Check sheet for the drawn part. Datum: minimum x, y, z corner. Units: mm. A direction names the side the tool comes from. Give positions to 0.01 mm unless a question says otherwise; leave off trailing zeros. Write each loop counter-clockwise with the first axis right and the second up, starting at its lowest first coordinate (ties: lowest second). Pieces come first, ordered by that corner, then holes. Notation, with made-up numbers: (66, -29) - (89, -29) arc R23 cw to (89, -14) - close; hole circle Ø9 at (6, 2). An arc over 180 degrees is marked (long way). Answer as a JSON object with one key per item and string values. Group by question number.
Item 1: Sectioned sample at A-A, the plane z = 16.5. Record the boundary of the cut face in (x, y).
Item 2: Sectioned sample at C-C, the plane z = 5.25. Record the boundary of the cut face in (x, y).
Item 3: Tool access check on the marked faces 1 and 2. Record the directions out of +Z, -Z, +X, -X, +Y, -Y that give a thin tool (end or side, any length) a straight path to the whole face; none if there is none.
Item 4: Draft check along Y on the marked faces 3, 4 and 5. Enter one of: +Y half, -Y half, draft (parallel to the pull), parting line (faces both ways), or undercut.
Item 5: Sectioned sample at B-B, the plane z = 9.5. Record the boundary of the cut face in (x, y).
Item 6: Go/stop test with flat-tipped pins: pin 1 (12 mm diameter, centred on x = 9.5, z = 3.5, fed in from -Y); pin 2 (12 mm diameter, centred on y = 35.5, z = 20.5, fed in from +X); pin 3 (1.5 mm diameter, centred on y = 30, z = 4, fed in from -X). Record where each tip stops, or that it passes through.
Item 7: Scan lines: line 1 along Y through (x, z) = (18.5, 19); line 2 along Y through (x, z) = (25, 20.5); line 3 along Z through (x, y) = (27.5, 6). Record each from-to range of solid material in increasing order. Write a range as [from, to].
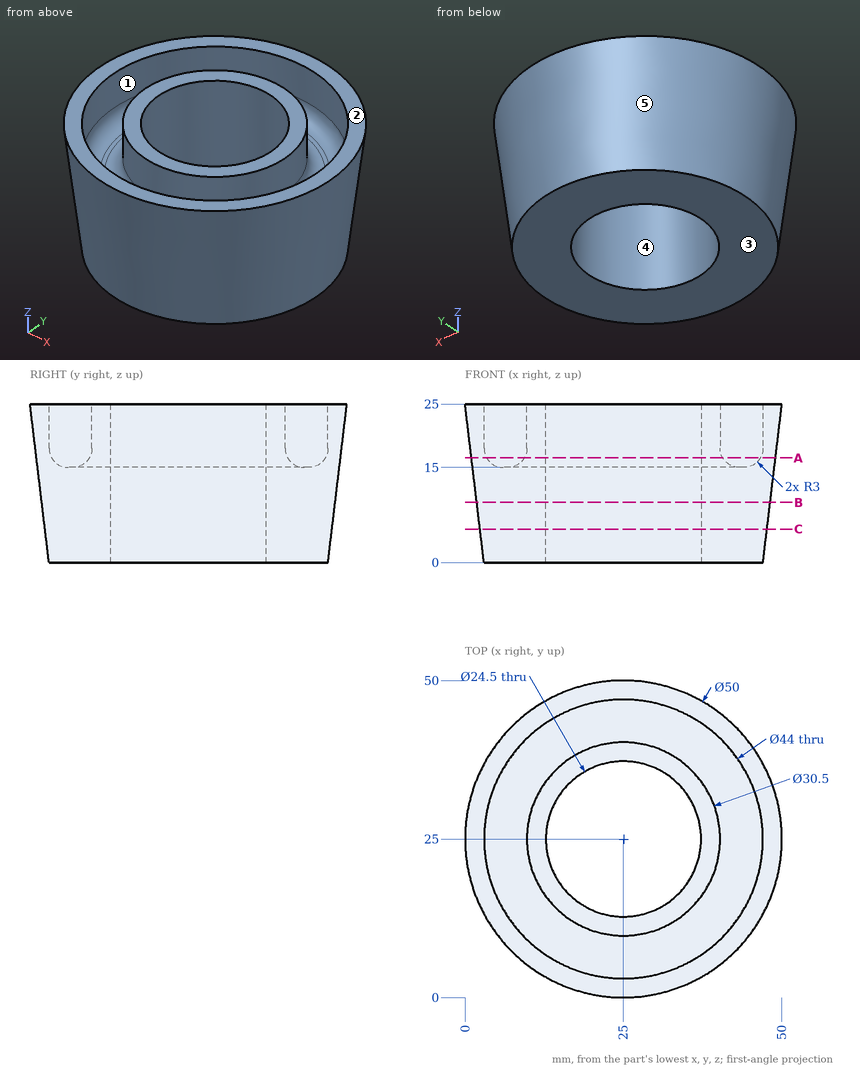
Geometry check:
{
 "1": {"outline": "circle Ø47.96 at (25, 25); circle Ø31.3 at (25, 25); hole circle Ø43.2 at (25, 25); hole circle Ø24.5 at (25, 25)"},
 "2": {"outline": "circle Ø45.26 at (25, 25); hole circle Ø24.5 at (25, 25)"},
 "3": {"face 1": "+Z", "face 2": "+Z, +X, -X, +Y, -Y"},
 "4": {"face 3": "draft", "face 4": "undercut", "face 5": "parting line"},
 "5": {"outline": "circle Ø46.28 at (25, 25); hole circle Ø24.5 at (25, 25)"},
 "6": {"pin 1": "y = 4.58", "pin 2": "x = 49.25", "pin 3": "x = 2.9"},
 "7": {"line 1": "[1.61, 3.98], [11.2, 14.62], [35.38, 38.8], [46.02, 48.39]", "line 2": "[0.54, 3], [9.75, 12.75], [37.25, 40.25], [47, 49.46]", "line 3": "[0, 15]"}
}
